For this review, take the finished solid that the model builds, in its own axes (mm). A direction names the side the tool comes from. Round coordinates to 2 decimals unless told otherwise and drop trailing zeros. Order: outer loops, then holes, each group sorted by start corner. A loop starts at its lowest first (then second) coordinate and runs counter-clockwise, first axis right, second up. Notation, with made-up numbers: (30, -23) -> (34, -23) arc R13 ccw to (34, -6) -> close; hole circle Ø8 at (-17, 49.25). An arc over 180 degrees is marked (long way). Use a Markdown table: item, result. Add a question column.
1) Consider section D-D (y = -1). State the section outline as (x, z) points.
2) Consider section B-B (x = 5). State the section outline as (y, z) points, plus the area to 3 significant figures.
3) Consider section A-A (y = -22.5). State the section outline as (x, z) points, plus the area to 3 significant figures.
4) Wall thickness on line 1 along Z through (x, y) = (0, 3.5) (3 decimals); line 2 along Y through (x, z) = (-6.5, -11); line 3 along Y through (x, z) = (2.5, -17): over which ranges is each line inside the solid? List them lowest first. Write a range as [from, to].
5) Machinability: for faces 5 (the face through (2.38, 2.96, 10.74)), 6 (the face through (-8, -4, 21)), which of the approach directions +Z, -Z, +X, -X, +Y, -Y give a long, thin tool a straight path to every point of the face, cutting with its end or side? Answer none if there is none.
6) Draft analysis for pull direction Y (two halves, no side actions). For faces 1 (the face through (-4.336, -42.024, 0.294)), 2 (the face through (2.976, 1.51, 2.282)), 3 (the face through (0, 6, -5)), 4 (the face through (0, -45, 5)), state which applies: pulls with the +Y half, pulls with the -Y half, needs draft (parallel to the pull), parting line crosses it, or undercut.
7) Clearance check with flat-ended pins moving along their axes: P1, Ø0.6, axis at x = 6.5, z = 0, coming from the +Y side; P2, Ø6, axis at x = 0, z = 16.5, coming from the +Y side. State where each tip first meets the part, or that it passes through.
8) Consider section C-C (z = 9). State the section outline as (x, y) points.
Autodesk Inventor part; units mm, degrees
ref_plane "YZ Plane" through (0, 0, 0) normal (1, 0, 0) x (0, 1, 0)
ref_plane "XZ Plane" through (0, 0, 0) normal (0, 1, 0) x (-1, 0, 0)
ref_plane "XY Plane" through (0, 0, 0) normal (0, 0, 1) x (1, 0, 0)
sketch "Sketch1" plane through (0, 0, 0) normal (0, 1, 0) x (-1, 0, 0)
  circle A0 centre (0, 0) radius 11
  circle A1 centre (0, 0) radius 3
  circle A2 centre (0, 0) radius 3.75
  circle A3 centre (0, 0) radius 6.375 construction
  circle A4 centre (0, 0) radius 9.375 construction
  circle A5 centre (0, 0) radius 7.875 construction
  circle A6 centre (0, -7.875) radius 0.35
  circle A7 centre (6.375, 0) radius 0.35
  circle A8 centre (9.375, 0) radius 0.35
  line L0 (16.292, 0) -> (-19, 0) construction
  line L1 (0, 21) -> (0, -27.3544) construction
  circle A9 centre (0, 7.875) radius 0.35
  circle A10 centre (-6.375, 0) radius 0.35
  circle A11 centre (-9.375, 0) radius 0.35
  line L2 (0, -21) -> (21, -21)
  line L3 (21, -21) -> (21, 0)
  line L4 (0, 21) -> (21, 21)
  line L5 (21, 21) -> (21, 0)
  line L6 (0, -21) -> (-21, -21)
  line L7 (-21, -21) -> (-21, 0)
  line L8 (-21, 21) -> (-21, 0)
  line L9 (0, 21) -> (-21, 21)
  dimension "d6" = 12.75
  dimension "d7" = 18.75
  dimension "d8" = 15.75
  dimension "d2" = 7.5
  dimension "d4" = 22
  dimension "d5" = 6
  dimension "d9" = 0.7
  dimension "d13" = 0.7
  dimension "d14" = 0.7
  dimension "d17" = 21
  dimension "d18" = 21
extrude "Extrusion1" add sketch "Sketch1" against normal blind 45 contours A0 | A6 | A7 | A8 | A9 | A10 | A11 | L6 L7 L8 L9 L4 L5 L3 L2
extrude "Extrusion2" add sketch "Sketch1" along normal blind 6 contours A0
sketch "Sketch2" plane through (-21, 0, 21) normal (0, 0, 1) x (1, 0, 0)
  line L0 (42, 0) -> (0, 0) construction
  line L1 (42, 0) -> (42, -45) construction
  line L2 (42, -45) -> (0, -45) construction
  line L3 (0, 0) -> (0, -45) construction
  line L4 (42, -45) -> (0, -45) construction
  line L5 (0, 0) -> (0, -45) construction
  line L6 (42, 0) -> (0, -45) construction
  line L7 (42, -45) -> (0, 0) construction
  circle A0 centre (21, -22.5) radius 20
  point P0 (21, 0)
  dimension "d23" = 40
extrude "Extrusion3" cut sketch "Sketch2" against normal blind 45
equation "\"d13\" = d9"
equation "\"d14\" = d9"
equation "\"d18\" = d17"
properties part number "engine_connector_sleeve"
Results list:
| question | item | result |
|---|---|---|
| 1 | outline | (-21, -21) -> (21, -21) -> (21, 21) -> (-21, 21) -> close; hole circle Ø7.5 at (0, 0) |
| 2 | outline | (-45, -21) -> (-41.86, -21) -> (-41.86, 21) -> (-45, 21) -> close; (-3.14, -21) -> (0, -21) -> (0, -9.8) -> (6, -9.8) -> (6, 9.8) -> (0, 9.8) -> (0, 21) -> (-3.14, 21) -> close |
| 2 | area | 381 mm2 |
| 3 | outline | (-21, -21) -> (-20, -21) -> (-20, 21) -> (-21, 21) -> close; (20, -21) -> (21, -21) -> (21, 21) -> (20, 21) -> close |
| 3 | area | 84.0 mm2 |
| 4 | line 1 | [-11, -8.225], [-7.525, -3.75], [3.75, 7.525], [8.225, 11] |
| 4 | line 2 | [-45, -41.41], [-3.59, 0] |
| 4 | line 3 | [-45, -42.34], [-2.66, 0] |
| 5 | face 5 | +Y |
| 5 | face 6 | +Z, +X, -X, +Y, -Y |
| 6 | face 1 | undercut |
| 6 | face 2 | needs draft |
| 6 | face 3 | pulls with the +Y half |
| 6 | face 4 | pulls with the -Y half |
| 7 | P1 | y = 6 |
| 7 | P2 | y = 0 |
| 8 | outline | (-21, -45) -> (21, -45) -> (21, 0) -> (6.32, 0) -> (6.32, 6) -> (-6.32, 6) -> (-6.32, 0) -> (-21, 0) -> close; hole circle Ø40 at (0, -22.5) |
